Verification items for the finished model (mm, model axes). A direction names the side the tool comes from. Give positions to 0.01 mm unless a question says otherwise; leave off trailing zeros. Order: outer loops, then holes, each group sorted by start corner. A loop starts at its lowest first (then second) coordinate and runs counter-clockwise, first axis right, second up.
from build123d import *

# Parameters (mm, degrees)
F0_W     = 150.821402669
F0_H     = 152.6858285069
F0_W_2   = 3.175
F0_H_2   = 25.4
F0_R     = 8.5350721602
F1_DEPTH = 5.08


with BuildPart() as f1:
    # F0 (on Top) → F1 (new body)
    with BuildSketch(Plane.XY):
        with Locations((-0.7561892271, -0.6262175739)):
            Rectangle(F0_W, F0_H)
        with Locations((-18.3173127979, -22.0731783986)):
            Rectangle(F0_W_2, F0_H_2, mode=Mode.SUBTRACT)
        with Locations((-31.1815738678, 57.5412772596)):
            Circle(F0_R, mode=Mode.SUBTRACT)
        with BuildLine():
            ThreePointArc((-2.437382494, 57.5412772596), (-11.2857981585, 48.6928615951), (-20.134213823, 57.5412772596))
            ThreePointArc((-20.134213823, 57.5412772596), (-11.2857981585, 66.3896929241), (-2.437382494, 57.5412772596))
        make_face(mode=Mode.SUBTRACT)
        with BuildLine():
            ThreePointArc((18.1603263455, 57.5412772596), (8.6099775508, 47.9909284649), (-0.9403712439, 57.5412772596))
            ThreePointArc((-0.9403712439, 57.5412772596), (8.6099775508, 67.0916260543), (18.1603263455, 57.5412772596))
        make_face(mode=Mode.SUBTRACT)
    extrude(amount=-F1_DEPTH)


solid = f1.part
(1) Section check B-B, the plane x = -31.5. Enter the section's corners in (y, z), then the cut area to 3 significant figures.
Solved:
outline: (-76.97, -5.08) - (49.01, -5.08) - (49.01, 0) - (-76.97, 0) - close; (66.07, -5.08) - (75.72, -5.08) - (75.72, 0) - (66.07, 0) - close
area: 689 mm2
(2) Section check D-D, the plane y = 60. Enter the section's corners in (x, z), then the cut area to 3 significant figures.
Solved:
outline: (-76.17, -5.08) - (-39.35, -5.08) - (-39.35, 0) - (-76.17, 0) - close; (-23.01, -5.08) - (-19.79, -5.08) - (-19.79, 0) - (-23.01, 0) - close; (-2.79, -5.08) - (-0.62, -5.08) - (-0.62, 0) - (-2.79, 0) - close; (17.84, -5.08) - (74.65, -5.08) - (74.65, 0) - (17.84, 0) - close
area: 503 mm2
(3) Section check A-A, the plane y = -22.5. Enter the section's corners in (x, z).
Solved:
outline: (-76.17, -5.08) - (-19.9, -5.08) - (-19.9, 0) - (-76.17, 0) - close; (-16.73, -5.08) - (74.65, -5.08) - (74.65, 0) - (-16.73, 0) - close
(4) Release check for a two-part mould opening along X. For faces 1 (the cylindrical face through (4.2, 49.07, -2.5)), 2 (the flat face through (-2, 0, 0)), 3 (the flat face through (-76.167, -2, -3)) record: pulls with the +X half, pulls with the -X half, needs draft (parallel to the pull), parting line crosses it, or undercut.
Solved:
face 1: undercut
face 2: needs draft
face 3: pulls with the -X half
(5) Set-up check for faces 4 (the flat face through (-16.73, -22, -3)), 5 (the flat face through (-2, 75.717, -3)): record each of +Z, -Z, +X, -X, +Y, -Y from which the full face is reachable in a straight line by a thin tool's end or side.
Solved:
face 4: +Z, -Z
face 5: +Z, -Z, +X, -X, +Y
(6) Section check C-C, the plane z = -1.75. Enter the section's corners in (x, y), then the cut area to 3 significant figures.
Solved:
outline: (-76.17, -76.97) - (74.65, -76.97) - (74.65, 75.72) - (-76.17, 75.72) - close; hole circle Ø17.07 at (-31.18, 57.54); hole circle Ø17.7 at (-11.29, 57.54); hole (-19.9, -34.77) - (-16.73, -34.77) - (-16.73, -9.37) - (-19.9, -9.37) - close; hole circle Ø19.1 at (8.61, 57.54)
area: 22,200 mm2
(7) Scan lines: line 1 (X direction, y = -10.5, z = -0.4); line 2 (X direction, y = 61.5, z = -2.6); line 3 (X direction, y = 65, z = -1.65). Record each from-to range of solid material in increasing order.
Solved:
line 1: x = -76.17 to -19.9, -16.73 to 74.65
line 2: x = -76.17 to -38.74, -23.62 to -19.2, -3.37 to -0.08, 17.3 to 74.65
line 3: x = -76.17 to -35.33, -27.03 to -16.05, -6.53 to 2.65, 14.57 to 74.65
